The model under review builds one solid part; all positions refer to its coordinate system, in mm. Face numbers are marked on the shaded views. Round coordinates to 2 decimals unless told otherwise and drop trailing zeros. Order: outer loops, then holes, each group sorted by start corner. A loop starts at its lowest first (then second) coordinate and runs counter-clockwise, first axis right, second up. Notation, with made-up numbers: M 71.25,16 L 99.25,16 A6 cw 99.25,20 Z; hole C 59,10 d11. An arc over 180 degrees is marked long. Answer as a JSON object with one key per item and string values. Group by question number.
1) To check wall thickness, follow line 1 (Y direction, x = -12.25, z = 88); line 2 (Z direction, x = -15, y = -18.5); line 3 (Z direction, x = -24, y = -40). State the ranges of each line that lie inside material, in increasing order.
2) Consider section C-C, the plane x = -2.75. Write out the cut boundary in (y, z).
3) Consider section A-A, the plane x = -19.5. Write out the cut boundary in (y, z), then the cut area to 3 significant figures.
4) Consider section D-D, the plane z = 80. Write out the cut boundary in (x, y).
5) Consider section B-B, the plane y = -7.5. Write out the cut boundary in (x, z), then the cut area to 3 significant figures.
6) The part is to be moulded in two halves that separate along Y. For the marked faces 1, 2 and 3, say which applies: +Y half, -Y half, draft (parallel to the pull), parting line (faces both ways), or undercut.
7) Insertion check: pin 1 Ø8.5 at (x, z) = (-17.5, 10) entering from -Y; pin 2 Ø1 at (x, z) = (-11, 81) entering from -Y; pin 3 Ø7 at (y, z) = (7.5, 52) entering from +X; pin 4 Ø6 at (x, y) = (-12.5, -24) entering from +Z. Each pin has a flat end and moves straight along its axis. Give the tip position at first contact, or say it passes through.
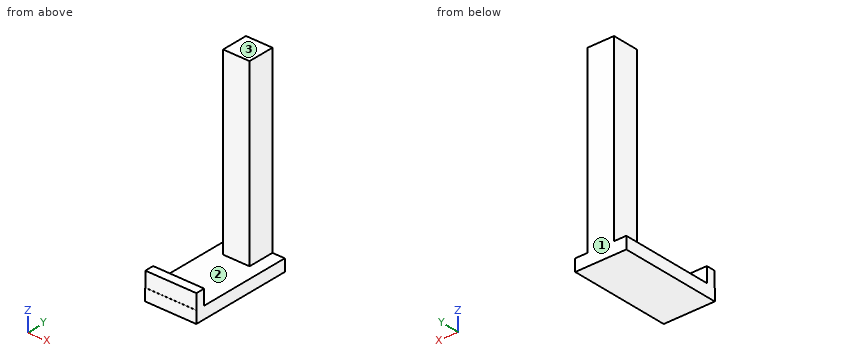
```python
from build123d import *

# Parameters (mm, degrees)
F0_W     = 26.9875
F0_H     = 53.975
F1_DEPTH = 6.35
F2_W     = 26.9875
F2_H     = 4.7625
F3_DEPTH = 7.9375
F4_W     = 6.985
F4_H     = 13.97
F5_DEPTH = 101.6


with BuildPart() as f1:
    # F0 (on Top) → F1 (new body)
    with BuildSketch(Plane.XY):
        with Locations((-13.6893766582, -15.4694584429)):
            Rectangle(F0_W, F0_H)
    extrude(amount=F1_DEPTH)

    # F2 (on face) → F3 (join)
    with BuildSketch(Plane.XY.offset(6.35)):
        with Locations((-13.6893766582, -40.0176870465)):
            Rectangle(F2_W, F2_H)
    extrude(amount=F3_DEPTH)

    # F4 (on Top) → F5 (join)
    with BuildSketch(Plane.XY):
        with Locations((-17.1818766582, 4.5330415571)):
            Rectangle(F4_W, F4_H)
        with Locations((-10.1968766582, 4.5330415571)):
            Rectangle(F4_W, F4_H)
    extrude(amount=F5_DEPTH)


solid = f1.part
```
Results list:
{
 "1": {"line 1": "-2.45 to 11.52", "line 2": "0 to 6.35", "line 3": "0 to 14.29"},
 "2": {"outline": "M -42.46,0 L 11.52,0 L 11.52,6.35 L -37.64,6.35 L -37.64,14.29 L -42.4,14.29 L -42.4,6.35 L -42.46,6.35 Z"},
 "3": {"outline": "M -42.46,0 L 11.52,0 L 11.52,101.6 L -2.45,101.6 L -2.45,6.35 L -37.64,6.35 L -37.64,14.29 L -42.4,14.29 L -42.4,6.35 L -42.46,6.35 Z", "area": "1,710 mm^2"},
 "4": {"outline": "M -20.67,-2.45 L -6.7,-2.45 L -6.7,11.52 L -20.67,11.52 Z"},
 "5": {"outline": "M -27.18,0 L -0.2,0 L -0.2,6.35 L -27.18,6.35 Z", "area": "171 mm^2"},
 "6": {"face 1": "+Y half", "face 2": "undercut", "face 3": "draft"},
 "7": {"pin 1": "y = -42.46", "pin 2": "y = -2.45", "pin 3": "x = -6.7", "pin 4": "z = 6.35"}
}
